```python
from build123d import *

# Parameters (mm, degrees)
SKETCH_1_R          = 2.75
EXTRUDE_1_DEPTH     = 3
CUT_EXTRUDE_1_DEPTH = 1.5
SKETCH_2_R          = 1.5
EXTRUDE_2_DEPTH     = 8
CHAMFER_1_SIZE      = 0.3
SCALE_1_SCALE       = 2


with BuildPart() as part:
    # 草图1 → 凸台-拉伸1 (new body)
    with BuildSketch(Plane(origin=(0, 0, 0), x_dir=(1, 0, 0), z_dir=(0, 1, 0))):
        with Locations(Location((0, 0, 0), (0, 0, 270))):
            Circle(SKETCH_1_R)
    extrude(amount=EXTRUDE_1_DEPTH)

    # 草图3 → 切除-拉伸1 (cut)
    with BuildSketch(Plane.XZ):
        Polygon((0, 1.25), (-1.082531755, 0.625), (-1.082531755, -0.625), (0, -1.25), (1.082531755, -0.625), (1.082531755, 0.625), align=None)
    extrude(amount=-CUT_EXTRUDE_1_DEPTH, mode=Mode.SUBTRACT)

    # 草图2 → 凸台-拉伸2 (add)
    with BuildSketch(Plane(origin=(0, 3, 0), x_dir=(1, 0, 0), z_dir=(0, 1, 0))):
        with Locations(Location((0, 0, 0), (0, 0, 270))):
            Circle(SKETCH_2_R)
    extrude(amount=EXTRUDE_2_DEPTH)

    # 倒角1
    chamfer_1_edges = [part.edges().sort_by_distance(p)[0] for p in [
        (0, 11, -1.5),
    ]]
    chamfer(chamfer_1_edges, length=CHAMFER_1_SIZE)


with BuildPart() as part_1:
    # 缩放比例1: scaled about (0, 4.07020226, 0)
    add(part.part.scale(SCALE_1_SCALE).moved(Location((0, -4.07020226, 0))))


solid = part_1.part
```
For this review, take the finished solid that the model builds, in its own axes (mm). A direction names the side the tool comes from. Round coordinates to 2 decimals unless told otherwise and drop trailing zeros. Write each loop counter-clockwise with the first axis right and the second up, starting at its lowest first coordinate (ties: lowest second). Pieces come first, ordered by that corner, then holes. Notation, with made-up numbers: (-21, 89.25) -> (-10, 89.25) arc R17 ccw to (-10, 95.25) -> close; hole circle Ø1 at (41.25, 32). An arc over 180 degrees is marked (long way). Use one line per item in the form item = value.
Q1. The part is to be moulded in two halves that separate along X. For faces 1 (the flat face through (-1.07, -2.59, 1.88)), 2 (the flat face through (-2.4, -4.07, -0.1)), 3 (the flat face through (-2.165, -3, 0)), 4 (the cylindrical face through (-5.37, -1.11, -1.19)), say which applies: released by +X, released by -X, zero draft, split by the parting line, or undercut.
Resolved:
face_1 = undercut
face_2 = zero draft
face_3 = undercut
face_4 = split by the parting line
Q2. Clearance check with flat-ended pins moving along their axes: pin 1 Ø4 at (x, y) = (1, 5) entering from +Z; pin 2 Ø2 at (x, y) = (-3.5, 9.5) entering from -Z; pin 3 Ø4 at (y, z) = (6, 3) entering from +X. State where each tip first meets the part, or that it passes through.
Resolved:
pin_1 = 3
pin_2 = -1.66
pin_3 = 2.83
Q3. Consider section A-A (y = -2.5). State the section outline as (x, z) points, then the cut area to 3 significant figures.
Resolved:
outline = circle Ø11 at (0, 0); hole (-2.17, -1.25) -> (0, -2.5) -> (2.17, -1.25) -> (2.17, 1.25) -> (0, 2.5) -> (-2.17, 1.25) -> close
area = 78.8 mm²
Q4. Consider section B-B (z = 0). State the section outline as (x, y) points, then the cut area to 3 significant figures.
Resolved:
outline = (-5.5, -4.07) -> (-2.17, -4.07) -> (-2.17, -1.07) -> (2.17, -1.07) -> (2.17, -4.07) -> (5.5, -4.07) -> (5.5, 1.93) -> (3, 1.93) -> (3, 17.33) -> (2.4, 17.93) -> (-2.4, 17.93) -> (-3, 17.33) -> (-3, 1.93) -> (-5.5, 1.93) -> close
area = 149 mm²
Q5. Machinability: for faces 5 (the flat face through (1.07, -2.59, -1.88)), 6 (the flat face through (-2.4, 1.93, 2.4)), 7 (the flat face through (0, 17.93, 0)), which of the approach directions +Z, -Z, +X, -X, +Y, -Y give a long, thin tool a straight path to every point of the face, cutting with its end or side? Answer none if there is none.
Resolved:
face_5 = -Y
face_6 = +Y
face_7 = +Z, -Z, +X, -X, +Y
Q6. Consider section D-D (x = -3.75). State the section outline as (y, z) points, then the cut area to 3 significant figures.
Resolved:
outline = (-4.07, -4.02) -> (1.93, -4.02) -> (1.93, 4.02) -> (-4.07, 4.02) -> close
area = 48.3 mm²
Q7. Consider section C-C (y = 9.5). State the section outline as (x, z) points, then the cut area to 3 significant figures.
Resolved:
outline = circle Ø6 at (0, 0)
area = 28.3 mm²
Q8. To check wall thickness, follow probe 1 along X at (y, z) = (-1.75, -0.25); probe 2 along Y at (x, z) = (-1.25, 3.5); probe 3 along Y at (x, z) = (0, 0.75). State the ranges of each line that lie inside material, in increasing order. Write a range as from..to.
Resolved:
probe_1 = -5.49..-2.17, 2.17..5.49
probe_2 = -4.07..1.93
probe_3 = -1.07..17.93
